Build history of the part. All positions in model axes, mm. Give positions to 0.01 mm unless a question says otherwise; leave off trailing zeros. Order: outer loops, then holes, each group sorted by start corner. A loop starts at its lowest first (then second) coordinate and runs counter-clockwise, first axis right, second up. Notation, with made-up numbers: M 80.5,50 L 125.5,50 A23 ccw 125.5,58 Z; hole C -9.5,63.25 d11. An arc over 180 degrees is marked long. One line per item, written item: value.
from build123d import *

# Parameters (mm, degrees)
BOSS_EXTRUDE1_DEPTH      = 6.35
BOSS_EXTRUDE1_DEPTH_BACK = 6.35
BOSS_EXTRUDE2_DEPTH      = 47.625
BOSS_EXTRUDE2_DEPTH_BACK = 60.325
SKETCH3_R                = 3.175
BOSS_EXTRUDE3_DEPTH      = 6.35
SKETCH5_R                = 9.525
BOSS_EXTRUDE4_DEPTH      = 3.175
SKETCH7_R                = 3.175
BOSS_EXTRUDE5_DEPTH      = 25.4


with BuildPart() as part:
    # Sketch2 → Boss-Extrude1 (new, two sides: drawn at the far end of the back side and taken through both)
    with BuildSketch(Plane(origin=(0, 0, 0), x_dir=(0, 0, -1), z_dir=(1, 0, 0)).offset(-BOSS_EXTRUDE1_DEPTH_BACK)):
        Polygon((4.171210262, -4.874787896), (6.307295287, 1.174980103), (2.136085025, 6.049767999), (-4.171210262, 4.874787896), (-6.307295287, -1.174980103), (-2.136085025, -6.049767999), align=None)
    extrude(amount=BOSS_EXTRUDE1_DEPTH + BOSS_EXTRUDE1_DEPTH_BACK)

    # Sketch3 → Boss-Extrude2 (add, two sides: drawn at the far end of the back side and taken through both)
    with BuildSketch(Plane(origin=(6.35, 0, 0), x_dir=(0, 0, -1), z_dir=(1, 0, 0)).offset(-BOSS_EXTRUDE2_DEPTH_BACK)):
        Circle(SKETCH3_R)
    extrude(amount=BOSS_EXTRUDE2_DEPTH + BOSS_EXTRUDE2_DEPTH_BACK)

    # Sketch4 → Boss-Extrude3 (add)
    with BuildSketch(Plane(origin=(53.975, 0, 0), x_dir=(0, 0, -1), z_dir=(1, 0, 0))):
        Polygon((4.488142835, -4.584662035), (6.214505208, 1.594514693), (1.726362373, 6.179176728), (-4.488142835, 4.584662035), (-6.214505208, -1.594514693), (-1.726362373, -6.179176728), align=None)
    boss_extrude3 = extrude(amount=BOSS_EXTRUDE3_DEPTH)

    # Sketch5 → Boss-Extrude4 (add)
    with BuildSketch(Plane(origin=(60.325, 0, 0), x_dir=(0, 0, -1), z_dir=(1, 0, 0))):
        Circle(SKETCH5_R)
    boss_extrude4 = extrude(amount=BOSS_EXTRUDE4_DEPTH)

    # Mirror1: Boss-Extrude3, Boss-Extrude4 across plane
    add(boss_extrude3.mirror(Plane(origin=(0, 0, 0), x_dir=(0, 0, 1), z_dir=(1, 0, 0))))
    add(boss_extrude4.mirror(Plane(origin=(0, 0, 0), x_dir=(0, 0, 1), z_dir=(1, 0, 0))))

    # Sketch7 → Boss-Extrude5 (add)
    with BuildSketch(Plane(origin=(63.5, 0, 0), x_dir=(0, 0, -1), z_dir=(1, 0, 0))):
        Circle(SKETCH7_R)
    boss_extrude5 = extrude(amount=BOSS_EXTRUDE5_DEPTH)

    # Mirror3: Boss-Extrude5 across plane
    add(boss_extrude5.mirror(Plane(origin=(0, 0, 0), x_dir=(0, 0, 1), z_dir=(1, 0, 0))))


solid = part.part
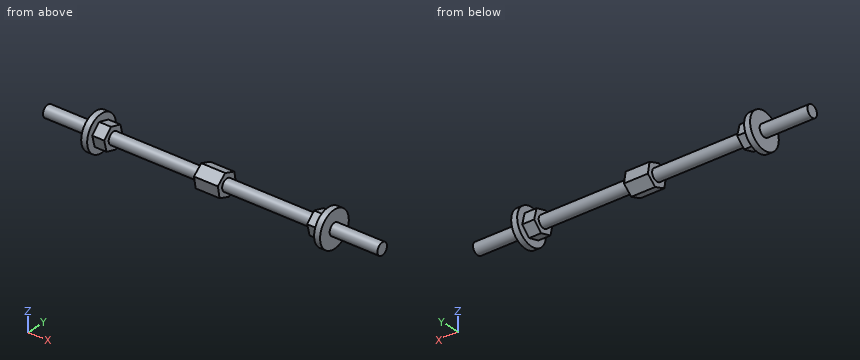
1) Saw through at A-A, the plane x = -70.5. Write the cut outline in (y, z) (3 decimals).
Check values:
outline: C 0,0 d6.35
2) Drill centre lines: probe 1 along X at (y, z) = (2.75, 2.25) (3 decimals); probe 2 along X at (y, z) = (-5.75, 4.5) (3 decimals); probe 3 along Y at (x, z) = (21.5, 0.25). Where is each one in solid material? Low to high. Write a range as from..to.
Check values:
probe 1: -63.5..-53.975, -6.35..6.35, 53.975..63.5
probe 2: -63.5..-60.325, 60.325..63.5
probe 3: -3.17..3.17
3) Pin check, flat tips, straight feed: pin 1 (1 mm diameter, centred on x = 63, y = -1, fed in from -Z); pin 2 (8 mm diameter, centred on x = -42.5, y = 7.5, fed in from -Z); pin 3 (6 mm diameter, centred on y = -6.5, z = -5.5, fed in from +X); pin 4 (10 mm diameter, centred on x = 54.5, z = -5.5, fed in from -Y). Stop position of each tip, or through.
Check values:
pin 1: z = -9.51
pin 2: through
pin 3: x = 63.5
pin 4: y = -5.61
